```python
from build123d import *

# Parameters (mm, degrees)
SKETCH1_R           = 15.875
BOSS_EXTRUDE1_DEPTH = 825.5
SKETCH2_R           = 22.711063055
SKETCH2_R_2         = 12.7
CUT_EXTRUDE1_DEPTH  = 127
CHAMFER1_SIZE       = 3.81


with BuildPart() as part:
    # Sketch1 → Boss-Extrude1 (new, symmetric)
    with BuildSketch(Plane.XY):
        Circle(SKETCH1_R)
    extrude(amount=BOSS_EXTRUDE1_DEPTH, both=True)

    # Sketch2 → Cut-Extrude1 (cut)
    with BuildSketch(Plane.XY.offset(825.5)):
        Circle(SKETCH2_R)
        Circle(SKETCH2_R_2, mode=Mode.SUBTRACT)
    cut_extrude1 = extrude(amount=-CUT_EXTRUDE1_DEPTH, mode=Mode.SUBTRACT)

    # Mirror1: Cut-Extrude1 across plane
    add(cut_extrude1.mirror(Plane.XY), mode=Mode.SUBTRACT)

    # Chamfer1
    # the kernel refuses this chamfer: 3.81 mm, written as the material it takes off along each edge
    with BuildSketch(Plane(origin=(0, 0, -698.5), x_dir=(1, 0, 0), z_dir=(0, -1, 0))) as chamfer1_piece_1_section:
        Polygon((15.875, CHAMFER1_SIZE), (15.875 - CHAMFER1_SIZE, 0), (15.875, 0), align=None)
    chamfer1_piece_1 = revolve(axis=Axis((0, 0, -698.5), (0, 0, 1)), mode=Mode.PRIVATE)
    chamfer1_piece_1 = chamfer1_piece_1 - Plane(origin=(0, 0, -696.286679129), x_dir=(1, 0, 0), z_dir=(0, 0, -1)) * Cylinder(12.7, 64, mode=Mode.PRIVATE)
    add(chamfer1_piece_1, mode=Mode.SUBTRACT)
    with BuildSketch(Plane(origin=(0, 0, 698.5), x_dir=(1, 0, 0), z_dir=(0, -1, 0))) as chamfer1_piece_2_section:
        Polygon((15.875, -CHAMFER1_SIZE), (15.875 - CHAMFER1_SIZE, 0), (15.875, 0), align=None)
    chamfer1_piece_2 = revolve(axis=Axis((0, 0, 698.5), (0, 0, 1)), mode=Mode.PRIVATE)
    chamfer1_piece_2 = chamfer1_piece_2 - Plane(origin=(0, 0, 696.286679129), x_dir=(1, 0, 0), z_dir=(0, 0, 1)) * Cylinder(12.7, 64, mode=Mode.PRIVATE)
    add(chamfer1_piece_2, mode=Mode.SUBTRACT)


solid = part.part
```
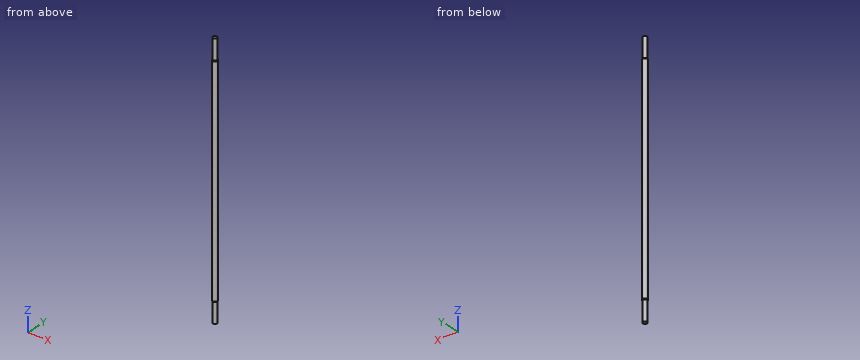
The listing builds one solid part. Answer for the finished solid, in the listing's coordinates (mm). Round coordinates to 2 decimals unless told otherwise and drop trailing zeros. Loops run counter-clockwise (first coordinate to the right, second up) from the corner with the lowest first, then second, coordinate; pieces in that order, holes last.
Q1. Section A-A, the plane y = 0 is taken. Determine the outline of the cut face in (x, z) (3 decimals), then the cut area to 3 significant figures.
Q2. Given pin 1 Ø4 at (x, y) = (12.5, -10) entering from -Z; pin 2 Ø1.5 at (x, z) = (6.5, 95) entering from +Y; pin 3 Ø6 at (x, z) = (-8.5, -471) entering from -Y, each flat-ended and moving along its own axis, determine where each tip first touches the part or whether it passes through.
Q3. Section C-C, the plane z = 580.5 is taken. Determine the outline of the cut face in (x, y) (3 decimals), then the cut area to 3 significant figures.
Q4. Find the intervals of material crossed by line 1 (X direction, y = 0.5, z = -652); line 2 (X direction, y = -9.5, z = 381); line 3 (Y direction, x = -4, z = 212), in increasing order.
Completed:
1. outline: (-15.875, -694.69) - (-12.7, -697.865) - (-12.7, -825.5) - (12.7, -825.5) - (12.7, -697.865) - (15.875, -694.69) - (15.875, 694.69) - (12.7, 697.865) - (12.7, 825.5) - (-12.7, 825.5) - (-12.7, 697.865) - (-15.875, 694.69) - close
1. area: 50,800 mm2
2. pin 1: stops at z = -696.56
2. pin 2: stops at y = 14.8
2. pin 3: stops at y = -14.89
3. outline: circle Ø31.75 at (0, 0)
3. area: 792 mm2
4. line 1: x = -15.87 to 15.87
4. line 2: x = -12.72 to 12.72
4. line 3: y = -15.36 to 15.36
